Autodesk Inventor part; units mm, degrees
ref_plane "Plano de trabajo1" through (0, 50, 30) normal (1, 0, 0) x (0, 0, -1)
ref_plane "Plano de trabajo2" through (-20, 50, 0) normal (0, 0, 1) x (1, 0, 0)
ref_plane "YZ Plane" through (0, 0, 0) normal (1, 0, 0) x (0, 1, 0)
sketch "Boceto1" plane through (0, 0, 0) normal (0, 1, 0) x (-1, 0, 0)
  circle A0 centre (0, 0) radius 15
  dimension "d0" = 30
extrude "Extrusión1" add sketch "Boceto1" along normal blind 50
sketch "Boceto2" plane through (0, 50, 0) normal (0, 1, 0) x (1, 0, 0)
  line L0 (20, 30) -> (-20, 30)
  line L1 (-20, 30) -> (-20, -30)
  line L2 (-20, -30) -> (20, -30)
  line L3 (20, -30) -> (20, 30)
  line L4 (20, 30) -> (-20, -30) construction
  line L5 (-20, 30) -> (20, -30) construction
  point P0 (0, 0)
  dimension "d3" = 60
  dimension "d4" = 40
extrude "Extrusión2" add sketch "Boceto2" along normal blind 5
sketch "Boceto3" plane through (-20, 50, 30) normal (0, 0, 1) x (1, 0, 0)
  line L0 (0, 5) -> (0, 25)
  line L1 (40, 5) -> (0, 5)
  line L2 (40, 5) -> (40, 25)
  arc A0 (40, 25) -> (0, 25) centre (20, 25) ccw
  circle A1 centre (20, 25) radius 5
  point P0 (20, -50)
  dimension "d7" = 20
  dimension "d8" = 20
  dimension "d9" = 10
extrude "Extrusión3" add sketch "Boceto3" against normal blind 5
sketch "Boceto4" plane through (20, 50, -30) normal (0, 0, -1) x (-1, 0, 0)
  circle A0 centre (20, 25) radius 5
  arc A1 (40, 25) -> (0, 25) centre (20, 25) ccw
  line L0 (40, 5) -> (40, 25)
  line L1 (0, 5) -> (40, 5)
  line L2 (0, 25) -> (0, 5)
  point P0 (20, -50)
extrude "Extrusión4" add sketch "Boceto4" against normal blind 5
sketch "Boceto5" plane through (20, 50, 30) normal (1, 0, 0) x (0, 0, -1)
  point P0 (30, -50)
ref_plane "Plano de trabajo1" through (0, 50, 30) normal (1, 0, 0) x (0, 0, -1)
ref_plane "Plano de trabajo2" through (-20, 50, 0) normal (0, 0, 1) x (1, 0, 0)
sketch "Boceto6" plane through (0, 50, 30) normal (1, 0, 0) x (0, 0, -1)
  line L0 (5, 25) -> (5, 45)
  line L1 (55, 7) -> (5, 7)
  line L2 (5, 7) -> (5, 45)
  line L3 (5, 45) -> (55, 45)
  line L4 (55, 45) -> (55, 7)
  line L5 (55, 7) -> (5, 45) construction
  line L6 (5, 7) -> (55, 45) construction
  point P0 (30, -50)
  point P1 (30, 26)
extrude "Extrusión5" add sketch "Boceto6" along normal mid plane 120
sketch "Boceto7" plane through (20, 50, -30) normal (0, 0, -1) x (-1, 0, 0)
  circle A0 centre (20, 25) radius 5
  point P0 (20, -50)
extrude "Extrusión6" cut sketch "Boceto7" against normal up to next
sketch "Boceto8" plane through (60, 50, 30) normal (1, 0, 0) x (0, 0, -1)
  line L0 (55, 7) -> (55, 5)
  line L1 (55, 7) -> (60, 7)
  line L2 (60, 7) -> (60, 107)
  line L3 (0, 7) -> (0, 107)
  line L4 (0, 107) -> (60, 107)
  line L5 (5, 25) -> (5, 7)
  line L6 (0, 7) -> (5, 7)
  line L7 (5, 7) -> (5, 45)
  line L8 (55, 45) -> (5, 45)
  line L9 (5, 45) -> (55, 45)
  line L10 (55, 45) -> (55, 7)
  point P0 (30, -50)
  dimension "d23" = 100
extrude "Extrusión7" add sketch "Boceto8" against normal blind 20
sketch "Boceto9" plane through (60, 57, -30) normal (0, 0, -1) x (-1, 0, 0)
  circle A0 centre (10, 18) radius 5
  point P0 (60, -57)
  dimension "d27" = 10
extrude "Extrusión8" cut sketch "Boceto9" against normal up to next
sketch "Boceto10" plane through (-60, 50, 30) normal (-1, 0, 0) x (0, 0, 1)
  line L0 (-60, 107) -> (-60, 7)
  line L1 (-5, 45) -> (-55, 45)
  line L2 (0, 107) -> (-60, 107)
  line L3 (-60, 7) -> (-55, 7)
  line L4 (-55, 45) -> (-55, 7)
  line L5 (-5, 45) -> (-55, 45)
  line L6 (-5, 7) -> (-5, 45)
  line L7 (-5, 7) -> (0, 7)
  line L8 (0, 7) -> (0, 107)
  line L9 (0, 107) -> (-60, 107)
  line L10 (-60, 107) -> (-60, 7)
  point P0 (-30, -50)
extrude "Extrusión9" add sketch "Boceto10" against normal blind 20
sketch "Boceto11" plane through (-60, 57, 30) normal (0, 0, 1) x (1, 0, 0)
  circle A0 centre (10, 18) radius 5
  point P0 (60, -57)
  dimension "d33" = 10
extrude "Extrusión10" cut sketch "Boceto11" against normal up to next
properties part number "pinza"
Could you check a few things on this model? Use its own coordinates, in mm. A direction names the side the tool comes from. Give positions to 0.01 mm unless a question says otherwise; leave off trailing zeros. Order: outer loops, then holes, each group sorted by start corner. A loop starts at its lowest first (then second) coordinate and runs counter-clockwise, first axis right, second up. Notation, with made-up numbers: (59.5, 57) - (85.5, 57) arc R5 ccw to (85.5, 64) - close; hole circle Ø11 at (-1.5, 23.25). An arc over 180 degrees is marked (long way). One line per item, written item: value. Start each with the question number.
1. For faces 1 (the face through (0, 95, 28)), 2 (the face through (-60, 108, 0)), 3 (the face through (29, 76, -25)), 4 (the face through (0, 68, 30)), 5 (the face through (20, 54, 0)), which set-ups out of +Z, -Z, +X, -X, +Y, -Y let a thin tool reach every point of the face, with its end or its side?
2. Imagine slicing it at D-D on x = -28. List the corners of the cut face in (y, z) for me.
3. Imagine slicing it at A-A on x = 50. List the corners of the cut face in (y, z) for me, plus the area to 3 significant figures.
4. For P1, Ø12, axis at y = 29.5, z = 13, coming from the +X side; P2, Ø20, axis at x = 9.5, z = -7, coming from the +Y side; P3, Ø6, axis at y = 41.5, z = -5, coming from the +X side, each with a flat end and sliding along its axis, tell me the tip position at first contact or that it passes through.
5. Imagine slicing it at C-C on z = 10. List the corners of the cut face in (x, y) for me, plus the area to 3 significant figures.
6. Imagine slicing it at B-B on z = 0. List the corners of the cut face in (x, y) for me, plus the area to 3 significant figures.
7. Thinking about a two-plate mould opening in Z: for faces 6 (the face through (0, 55, 0)), 7 (the face through (-1, 95, 0)), 8 (the face through (50, 106, 30)), which applies, +Z half, -Z half, draft (parallel to the pull), parting line (faces both ways), or undercut?
8. If I drill on probe 1 along Y at (x, z) = (0, -10); probe 2 along Y at (x, z) = (-50, 12); probe 3 along Y at (x, z) = (9, -17.5), over which ranges is the centre line in solid material (lowest first)?
Values:
1. face 1: +Z, +Y
1. face 2: +Z, -Z, -X, +Y, -Y
1. face 3: -Z, +Y
1. face 4: +Z, +X, -X, +Y, -Y
1. face 5: -Y
2. outline: (57, -25) - (95, -25) - (95, 25) - (57, 25) - close
3. outline: (57, -30) - (70, -30) - (70, 30) - (57, 30) - close; (80, -30) - (157, -30) - (157, 30) - (80, 30) - close
3. area: 5,400 mm²
4. P1: x = 13.27
4. P2: y = 95
4. P3: x = 14.87
5. outline: (-60, 57) - (60, 57) - (60, 157) - (40, 157) - (40, 95) - (-40, 95) - (-40, 157) - (-60, 157) - close; (-20, 50) - (-11.18, 50) - (-11.18, 0) - (11.18, 0) - (11.18, 50) - (20, 50) - (20, 55) - (-20, 55) - close; hole circle Ø10 at (-50, 75); hole circle Ø10 at (0, 75); hole circle Ø10 at (50, 75)
5. area: 8,120 mm²
6. outline: (-60, 57) - (60, 57) - (60, 157) - (40, 157) - (40, 95) - (-40, 95) - (-40, 157) - (-60, 157) - close; (-20, 50) - (-15, 50) - (-15, 0) - (15, 0) - (15, 50) - (20, 50) - (20, 55) - (-20, 55) - close; hole circle Ø10 at (-50, 75); hole circle Ø10 at (0, 75); hole circle Ø10 at (50, 75)
6. area: 8,500 mm²
7. face 6: undercut
7. face 7: draft
7. face 8: +Z half
8. probe 1: 0 to 55, 57 to 70, 80 to 95
8. probe 2: 57 to 70, 80 to 157
8. probe 3: 50 to 55, 57 to 95
